The listing builds one solid part. Answer for the finished solid, in the listing's coordinates (mm). Face numbers are marked on the shaded views. Round coordinates to 2 decimals unless told otherwise and drop trailing zeros. Write each loop counter-clockwise with the first axis right and the second up, starting at its lowest first coordinate (ties: lowest second). Pieces come first, ordered by that corner, then holes. Notation, with made-up numbers: (-3.5, -35.75) - (49.5, -35.75) arc R35 cw to (49.5, 1.25) - close; hole circle Ø8 at (-27.75, -14.75). An arc over 180 degrees is marked (long way). Answer as CSV lines item,"result". Start each with the question number.
Item 1: A cutting plane is placed at C-C on y = 16.75. Determine the outline of the cut face in (x, z).
Item 2: A cutting plane is placed at A-A on x = 71. Determine the outline of the cut face in (y, z).
Item 3: Straight lines are drawn through the part: line 1 along X through (y, z) = (1.5, -60.5); line 2 along X through (y, z) = (2.75, 3); line 3 along Y through (x, z) = (19, 46.5). For each, find the intervals that lie inside material, in ascending order. Write a range as [from, to].
Item 4: A cutting plane is placed at B-B on z = 47. Determine the outline of the cut face in (x, y), and give its area (3 significant figures).
Item 5: A flat-ended cylindrical pin translates along its axis: pin 1 (0.5 mm diameter, centred on x = -77.5, z = 81, fed in from -Y). Find the tip coordinate at first contact, or state that the pin passes through.
Item 6: For a pull along X with two mould halves and no side action, classify the marked faces 1 and 2 as pulls with the +X half, pulls with the -X half, needs draft (parallel to the pull), parting line crosses it, or undercut.
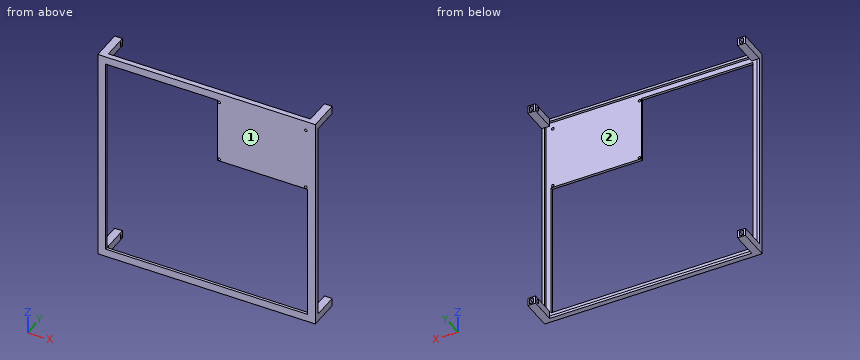
```python
from build123d import *

# Parameters (mm, degrees)
SKETCH1_W            = 164.3375
SKETCH1_H            = 164.3375
SKETCH1_R            = 1
BOSS_EXTRUDE1_DEPTH  = 2
SKETCH1_3_W          = 168.3375
SKETCH1_3_H          = 168.3375
SKETCH1_3_W_2        = 164.3375
SKETCH1_3_H_2        = 164.3375
BOSS_EXTRUDE2_DEPTH  = 4
SKETCH2_W            = 6
SKETCH2_H            = 6
BOSS_EXTRUDE3_DEPTH  = 20
SKETCH3_W            = 3
SKETCH3_H            = 4
CUT_EXTRUDE1_DEPTH   = 4
BOSS_EXTRUDE4_START  = -1.5
BOSS_EXTRUDE4_DEPTH  = 3
MIRROR2_START        = -1.5
MIRROR2_COPY_1_DEPTH = 3


with BuildPart() as part:
    # Sketch1 → Boss-Extrude1 (new body)
    with BuildSketch(Plane(origin=(0, 0, 0), x_dir=(1, 0, 0), z_dir=(0, 1, 0))):
        Rectangle(SKETCH1_W, SKETCH1_H)
        Polygon((8.31875, -27.36875), (8.31875, -78.16875), (-78.16875, -78.16875), (-78.16875, 78.16875), (78.16875, 78.16875), (78.16875, -27.36875), (9.71875, -27.36875), align=None, mode=Mode.SUBTRACT)
        with Locations(Location((9.71875, -76.76875, 0), (0, 0, 270))):
            Circle(SKETCH1_R, mode=Mode.SUBTRACT)
        with Locations(Location((76.76875, -76.76875, 0), (0, 0, 270))):
            Circle(SKETCH1_R, mode=Mode.SUBTRACT)
        with Locations(Location((9.71875, -28.76875, 0), (0, 0, 270))):
            Circle(SKETCH1_R, mode=Mode.SUBTRACT)
        with Locations(Location((76.76875, -28.76875, 0), (0, 0, 270))):
            Circle(SKETCH1_R, mode=Mode.SUBTRACT)
    extrude(amount=BOSS_EXTRUDE1_DEPTH)

    # Sketch1_3 → Boss-Extrude2 (add)
    with BuildSketch(Plane(origin=(0, 0, 0), x_dir=(1, 0, 0), z_dir=(0, 1, 0))):
        Rectangle(SKETCH1_3_W, SKETCH1_3_H)
        Rectangle(SKETCH1_3_W_2, SKETCH1_3_H_2, mode=Mode.SUBTRACT)
    extrude(amount=BOSS_EXTRUDE2_DEPTH)

    # Sketch2 → Boss-Extrude3 (add)
    with BuildSketch(Plane(origin=(0, 4, 0), x_dir=(1, 0, 0), z_dir=(0, 1, 0))):
        with Locations((-81.16875, 81.16875)):
            Rectangle(SKETCH2_W, SKETCH2_H)
        with Locations((81.16875, 81.16875)):
            Rectangle(SKETCH2_W, SKETCH2_H)
        with Locations((81.16875, -81.16875)):
            Rectangle(SKETCH2_W, SKETCH2_H)
        with Locations((-81.16875, -81.16875)):
            Rectangle(SKETCH2_W, SKETCH2_H)
    extrude(amount=BOSS_EXTRUDE3_DEPTH)

    # Sketch3 → Cut-Extrude1 (cut)
    with BuildSketch(Plane(origin=(0, 24, 0), x_dir=(1, 0, 0), z_dir=(0, 1, 0))):
        with Locations((81.16875, -81.16875)):
            Rectangle(SKETCH3_W, SKETCH3_H)
        with Locations((81.16875, 81.16875)):
            Rectangle(SKETCH3_W, SKETCH3_H)
        with Locations((-81.16875, 81.16875)):
            Rectangle(SKETCH3_W, SKETCH3_H)
        with Locations((-81.16875, -81.16875)):
            Rectangle(SKETCH3_W, SKETCH3_H)
    extrude(amount=-CUT_EXTRUDE1_DEPTH, mode=Mode.SUBTRACT)

    # Sketch4 → Boss-Extrude4 (add)
    with BuildSketch(Plane(origin=(0, 0, 78.16875), x_dir=(-1, 0, 0), z_dir=(0, 0, -1)).offset(BOSS_EXTRUDE4_START)):
        Polygon((-77.56875, 21), (-78.16875, 22), (-78.16875, 21), align=None)
    boss_extrude4 = extrude(amount=-BOSS_EXTRUDE4_DEPTH)

    # Mirror1: Boss-Extrude4 across plane
    add(boss_extrude4.mirror(Plane(origin=(0, 0, 0), x_dir=(0, 0, 1), z_dir=(1, 0, 0))))

    # Mirror2: Boss-Extrude4 across plane
    add(boss_extrude4.mirror(Plane.XY))

    # Mirror2 copy 1 sketch → Mirror2 copy 1 (add)
    with BuildSketch(Plane.XY.offset(-78.16875).offset(MIRROR2_START)):
        Polygon((-77.56875, 21), (-78.16875, 22), (-78.16875, 21), align=None)
    extrude(amount=-MIRROR2_COPY_1_DEPTH)


solid = part.part
```
Geometry says:
1,outline,"(-84.17, -84.17) - (-78.17, -84.17) - (-78.17, -78.17) - (-84.17, -78.17) - close; (-84.17, 78.17) - (-78.17, 78.17) - (-78.17, 84.17) - (-84.17, 84.17) - close; (78.17, -84.17) - (84.17, -84.17) - (84.17, -78.17) - (78.17, -78.17) - close; (78.17, 78.17) - (84.17, 78.17) - (84.17, 84.17) - (78.17, 84.17) - close"
2,outline,"(0, -84.17) - (4, -84.17) - (4, -82.17) - (2, -82.17) - (2, -78.17) - (0, -78.17) - close; (0, 27.37) - (2, 27.37) - (2, 82.17) - (4, 82.17) - (4, 84.17) - (0, 84.17) - close"
3,line 1,"x = [-84.17, -78.17], [78.17, 84.17]"
3,line 2,"x = [-84.17, -82.17], [82.17, 84.17]"
3,line 3,"y = [0, 2]"
4,outline,"(-84.17, 0) - (-78.17, 0) - (-78.17, 2) - (-82.17, 2) - (-82.17, 4) - (-84.17, 4) - close; (8.32, 0) - (84.17, 0) - (84.17, 4) - (82.17, 4) - (82.17, 2) - (8.32, 2) - close"
4,area,"172 mm^2"
5,pin 1,"stops at y = 0"
6,face 1,"needs draft"
6,face 2,"undercut"
